Read the model definition and answer for the solid it produces. Units are mm, in the model's axes. Face numbers are marked on the shaded views. A direction names the side the tool comes from. Coordinates: 2 decimals unless noted, no trailing zeros. Write each loop counter-clockwise with the first axis right and the second up, starting at its lowest first coordinate (ties: lowest second). Pieces come first, ordered by that corner, then holes. Notation, with made-up numbers: M 68,5 L 102,5 A13 cw 102,15 Z; hole C -14,-8.5 d1. An arc over 180 degrees is marked long. Use a Markdown table: item, result. Add a question column.
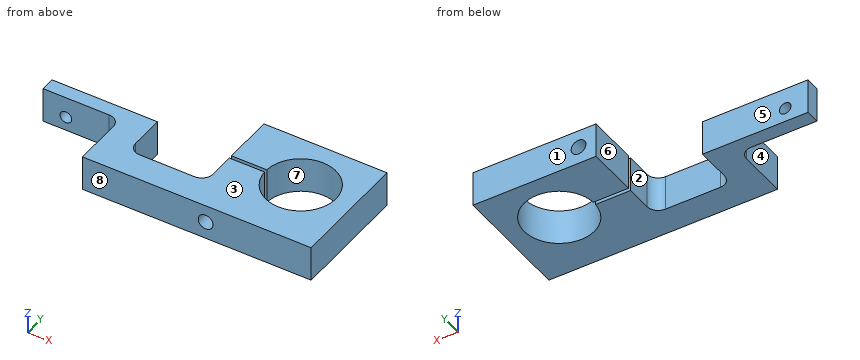
from build123d import *

# Parameters (mm, degrees)
F1_DEPTH = 10
F3_D     = 4.2
F5_D     = 3.3


with BuildPart() as f1:
    # F0 (on Top) → F1 (new body)
    with BuildSketch(Plane.XY):
        with BuildLine():
            ThreePointArc((-9.9874921777, 0.5), (10, 0), (-9.9874921777, -0.5))
            Line((-9.9874921777, -0.5), (-20, -0.5))
            Line((-20, -0.5), (-20, -7.825))
            ThreePointArc((-20, -7.825), (-20.9299359697, -10.0700640303), (-23.175, -11))
            Line((-23.175, -11), (-38.825, -11))
            ThreePointArc((-38.825, -11), (-41.0700640303, -10.0700640303), (-42, -7.825))
            Line((-42, -7.825), (-42, 2))
            Line((-42, 2), (-72, 2))
            Line((-72, 2), (-72, -2))
            Line((-72, -2), (-53.175, -2))
            ThreePointArc((-53.175, -2), (-50.9299359697, -2.9299359697), (-50, -5.175))
            Line((-50, -5.175), (-50, -19))
            Line((-50, -19), (15, -19))
            Line((15, -19), (15, 15))
            Line((15, 15), (-20, 15))
            Line((-20, 15), (-20, 0.5))
            Line((-20, 0.5), (-9.9874921777, 0.5))
        make_face()
    extrude(amount=F1_DEPTH)

    # F3 (through all)
    with Locations(Plane(origin=(0, 15, 0), x_dir=(-1, 0, 0), z_dir=(0, 1, 0))):
        with Locations((15, 5)):
            Hole(F3_D / 2)

    # F5 (through all)
    with Locations(Plane(origin=(0, 2, 0), x_dir=(-1, 0, 0), z_dir=(0, 1, 0))):
        with Locations((65.5, 4)):
            Hole(F5_D / 2)


solid = f1.part
Item 1: Each of these flat-tipped pins is pushed along its axis until it touches: pin 1 (5 mm diameter, centred on x = -61.5, z = 7, fed in from +Y); pin 2 (5 mm diameter, centred on y = -9, z = 7.5, fed in from -X). Where does it stop, or does it pass through?
Item 2: Find section C-C on x = -15. Give the vertices of the cut face in (y, z).
Item 3: Find section A-A on x = -65.5. Give the vertices of the cut face in (y, z), then the cut area to 3 significant figures.
Item 4: Find section B-B on y = 7. Give the vertices of the cut face in (x, z), then the cut area to 3 significant figures.
Item 5: Determine the mould class of the marked faces 6, 7 and 8 for opening direction Y: pulls with the +Y half, pulls with the -Y half, needs draft (parallel to the pull), parting line crosses it, or undercut.
Item 6: Consider probe 1 along Y at (x, z) = (-13.5, 7.75); probe 2 along Z at (x, y) = (-15, -7); probe 3 along Y at (x, z) = (0, 5.5). Determine where each line is inside the solid, lowest interval first.
Item 7: For the marked faces 1, 2, 3, 4 and 5, determine the directions among +Z, -Z, +X, -X, +Y, -Y from which every point of the face is accessible in a straight line to the end or side of a thin tool.
Geometry says:
| question | item | result |
|---|---|---|
| 1 | pin 1 | stops at y = 2 |
| 1 | pin 2 | stops at x = -50 |
| 2 | outline | M -19,0 L -0.5,0 L -0.5,2.9 L -19,2.9 Z; M -19,7.1 L -0.5,7.1 L -0.5,10 L -19,10 Z; M 0.5,0 L 15,0 L 15,2.9 L 0.5,2.9 Z; M 0.5,7.1 L 15,7.1 L 15,10 L 0.5,10 Z |
| 3 | outline | M -2,0 L 2,0 L 2,2.35 L -2,2.35 Z; M -2,5.65 L 2,5.65 L 2,10 L -2,10 Z |
| 3 | area | 26.8 mm2 |
| 4 | outline | M -20,0 L -7.14,0 L -7.14,10 L -20,10 Z; M 7.14,0 L 15,0 L 15,10 L 7.14,10 Z; hole C -15,5 d4.2 |
| 4 | area | 193 mm2 |
| 5 | face 6 | needs draft |
| 5 | face 7 | undercut |
| 5 | face 8 | pulls with the -Y half |
| 6 | probe 1 | y = -19 to -0.5, 0.5 to 15 |
| 6 | probe 2 | z = 0 to 2.9, 7.1 to 10 |
| 6 | probe 3 | y = -19 to -10, 10 to 15 |
| 7 | face 1 | +Z, -Z, +X, -X, +Y |
| 7 | face 2 | +Z, -Z, +Y |
| 7 | face 3 | +Z, +X, -X, +Y, -Y |
| 7 | face 4 | +Z, -Z, -X, -Y |
| 7 | face 5 | +Z, -Z, -X, +Y |
